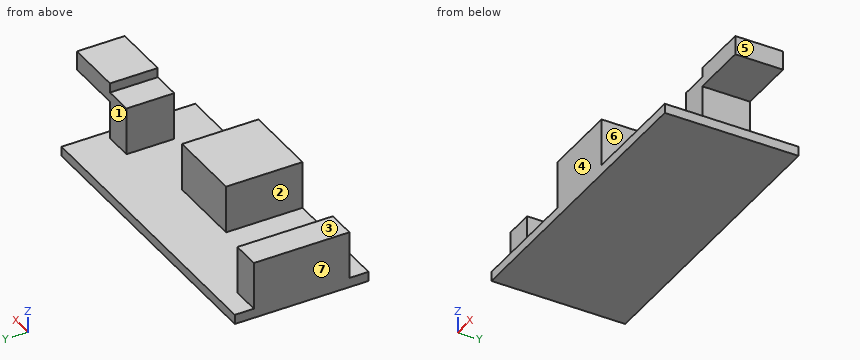
from build123d import *

# Parameters (mm, degrees)
ESQUISSE1_W        = 31.5
ESQUISSE1_H        = 14
BOSS_EXTRU_1_DEPTH = 1
ESQUISSE2_W        = 8
ESQUISSE2_H        = 8
BOSS_EXTRU_2_DEPTH = 5
ESQUISSE3_W        = 3
ESQUISSE3_H        = 5
BOSS_EXTRU_3_DEPTH = 5
ESQUISSE4_W        = 3
ESQUISSE4_H        = 10
BOSS_EXTRU_4_DEPTH = 5
ESQUISSE6_W        = 2
ESQUISSE6_H        = 5
BOSS_EXTRU_6_DEPTH = 6


with BuildPart() as part:
    # Esquisse1 → Boss.-Extru.1 (new body)
    with BuildSketch(Plane.XY):
        with Locations((-3.425842613, 1.088280058)):
            Rectangle(ESQUISSE1_W, ESQUISSE1_H)
    extrude(amount=-BOSS_EXTRU_1_DEPTH)

    # Esquisse2 → Boss.-Extru.2 (add)
    with BuildSketch(Plane.XY):
        with Locations((-3.175842613, -1.911719942)):
            Rectangle(ESQUISSE2_W, ESQUISSE2_H)
    extrude(amount=BOSS_EXTRU_2_DEPTH)

    # Esquisse3 → Boss.-Extru.3 (add)
    with BuildSketch(Plane.XY):
        with Locations((9.824157387, 1.088280058)):
            Rectangle(ESQUISSE3_W, ESQUISSE3_H)
    extrude(amount=BOSS_EXTRU_3_DEPTH)

    # Esquisse4 → Boss.-Extru.4 (add)
    with BuildSketch(Plane.XY):
        with Locations((-17.675842613, 1.088280058)):
            Rectangle(ESQUISSE4_W, ESQUISSE4_H)
    extrude(amount=BOSS_EXTRU_4_DEPTH)

    # Esquisse6 → Boss.-Extru.6 (add)
    with BuildSketch(Plane(origin=(11.324157387, 0, 0), x_dir=(0, 0, -1), z_dir=(1, 0, 0))):
        with Locations((-5, 1.088280058)):
            Rectangle(ESQUISSE6_W, ESQUISSE6_H)
    extrude(amount=BOSS_EXTRU_6_DEPTH)


solid = part.part
Geometry check sheet. Reference: the model listing, model coordinates, mm. Face numbers are marked on the shaded views. A direction names the side the tool comes from. Give positions to 0.01 mm unless a question says otherwise; leave off trailing zeros. Order: outer loops, then holes, each group sorted by start corner. A loop starts at its lowest first (then second) coordinate and runs counter-clockwise, first axis right, second up.
1) Tool access check on the marked faces 1, 2 and 3. Record the directions out of +Z, -Z, +X, -X, +Y, -Y that give a thin tool (end or side, any length) a straight path to the whole face; none if there is none.
Results are:
face 1: +Z, +X, +Y
face 2: +Z, +Y, -Y
face 3: +Z, -X, +Y, -Y
2) Draft check along X on the marked faces 4, 5, 6 and 7. Enter one of: released by +X, released by -X, zero draft, split by the parting line, or undercut.
Results are:
face 4: zero draft
face 5: released by +X
face 6: undercut
face 7: released by -X
3) Cross-section at C-C (z = 5.5). Record the boundary of the cut face in (x, y).
Results are:
outline: (11.32, -1.41) - (17.32, -1.41) - (17.32, 3.59) - (11.32, 3.59) - close
4) Cross-section at B-B (y = 1.5). Record the boundary of the cut face in (x, z).
Results are:
outline: (-19.18, -1) - (12.32, -1) - (12.32, 0) - (11.32, 0) - (11.32, 4) - (17.32, 4) - (17.32, 6) - (11.32, 6) - (11.32, 5) - (8.32, 5) - (8.32, 0) - (0.82, 0) - (0.82, 5) - (-7.18, 5) - (-7.18, 0) - (-16.18, 0) - (-16.18, 5) - (-19.18, 5) - close
5) Cross-section at D-D (y = 5.75). Record the boundary of the cut face in (x, z), then the cut area to 3 significant figures.
Results are:
outline: (-19.18, -1) - (12.32, -1) - (12.32, 0) - (-16.18, 0) - (-16.18, 5) - (-19.18, 5) - close
area: 46.5 mm2
6) Material ranges on probe 1 along X at (y, z) = (-0.75, 3.25); probe 2 along X at (y, z) = (-2.5, 4.5); probe 3 along X at (y, z) = (3.5, 3.75), recorded low to high.
Results are:
probe 1: x = -19.18 to -16.18, -7.18 to 0.82, 8.32 to 11.32
probe 2: x = -19.18 to -16.18, -7.18 to 0.82
probe 3: x = -19.18 to -16.18, 8.32 to 11.32
7) Cross-section at A-A (x = -2). Record the boundary of the cut face in (y, z).
Results are:
outline: (-5.91, -1) - (8.09, -1) - (8.09, 0) - (2.09, 0) - (2.09, 5) - (-5.91, 5) - close
8) Gauge pin test, flat ends, axial feed: pin 1 (2.5 mm diameter, centred on x = -1.5, z = 2, fed in from +Y); pin 2 (0.8 mm diameter, centred on y = 4.5, z = -0.5, fed in from +X); pin 3 (0.9 mm diameter, centred on x = -17, y = -1.5, fed in from +Z). Record the tip position at first contact, or that the pin passes through.
Results are:
pin 1: stops at y = 2.09
pin 2: stops at x = 12.32
pin 3: stops at z = 5
